from build123d import *

# Parameters (mm, degrees)
SKETCH016_R            = 4.25
PAD015_DEPTH           = 30
PAD014_DEPTH           = 3
PRISM008_DEPTH         = 10
PRISM008_ROLL_ANGLE    = 90
PAD011_DEPTH           = 15
SKETCH010_R            = 1
PAD010_DEPTH           = 22.5
CYLINDER017_R          = 4.25
CYLINDER017_DEPTH      = 10
CYLINDER016_R          = 5.25
CYLINDER016_DEPTH      = 10
CYLINDER014_R          = 1.75
CYLINDER014_DEPTH      = 36
CYLINDER014_ROLL_ANGLE = -90
PAD004_DEPTH           = 5
CHAMFER002_SIZE        = 1
CYLINDER012_R          = 1.75
CYLINDER012_DEPTH      = 11
CYLINDER012_ROLL_ANGLE = 90
CYLINDER013_R          = 5.5
CYLINDER013_DEPTH      = 14
CYLINDER013_ROLL_ANGLE = -90
BOX010_W               = 35
BOX010_H               = 60
BOX010_DEPTH           = 35
PAD003_DEPTH           = 42
FILLET002_R            = 0.5
CHAMFER003_SIZE        = 1
CHAMFER006_SIZE        = 2
CHAMFER007_SIZE        = 1


with BuildPart() as pad015:
    # Sketch016 → Pad015 (new body)
    with BuildSketch(Plane(origin=(23.25, 34, -10), x_dir=(-0.996195, -0.087156, 0), z_dir=(0, 0, 1))):
        with Locations((47, 7)):
            Circle(SKETCH016_R)
    extrude(amount=PAD015_DEPTH)


with BuildPart() as fusion011:
    # Sketch014 → Pad014 (new body)
    with BuildSketch(Plane(origin=(23.25, 34, -10), x_dir=(-0.996195, -0.087156, 0), z_dir=(0, 0, 1))):
        with BuildLine():
            ThreePointArc((49.709474, 10.274332), (43.52198, 9.442514), (44.839693, 3.340003))
            Line((44.839693, 3.340003), (61.15095, -6.287705))
            ThreePointArc((61.15095, -6.287705), (64.799282, -5.499923), (64.301984, -1.800786))
            Line((49.709474, 10.274332), (64.301984, -1.800786))
        make_face()
    extrude(amount=PAD014_DEPTH)

    # Fusion011: union Pad015
    add(pad015.part)


with BuildPart() as fake_axis_nut_room:
    # Prism008 → Prism008 (new body)
    with BuildSketch(Plane.XY):
        Polygon((3.2, 0), (1.6, 2.771281), (-1.6, 2.771281), (-3.2, 0), (-1.6, -2.771281), (1.6, -2.771281), align=None)
    extrude(amount=PRISM008_DEPTH)


with BuildPart() as fake_axis_nut_room_1:
    # Prism008 roll: moved
    add(fake_axis_nut_room.part.rotate(Axis((0, 0, 0), (1, 0, 0)), PRISM008_ROLL_ANGLE))


with BuildPart() as fake_axis_nut_room_2:
    # Prism008 placement: moved
    add(fake_axis_nut_room_1.part.moved(Location((-47, 25.5, 7))))


with BuildPart() as pad011:
    # Sketch011 → Pad011 (new body)
    with BuildSketch(Plane(origin=(0, 0, -10), x_dir=(1, 0, 0), z_dir=(0, 0, -1))):
        with BuildLine():
            ThreePointArc((-48.5, -22.8), (-50.7, -25), (-48.5, -27.2))
            Line((-48.5, -27.2), (-39.5, -27.2))
            ThreePointArc((-39.5, -27.2), (-37.3, -25), (-39.5, -22.8))
            Line((-48.5, -22.8), (-39.5, -22.8))
        make_face()
    extrude(amount=-PAD011_DEPTH)


with BuildPart() as pad010:
    # Sketch010 → Pad010 (new body)
    with BuildSketch(Plane(origin=(0, 41, 0), x_dir=(-1, 0, 0), z_dir=(0, 1, 0))):
        with Locations((43.25, 26.75)):
            Circle(SKETCH010_R)
        with Locations((50.75, 26.75)):
            Circle(SKETCH010_R)
        with Locations((43.25, -1.25)):
            Circle(SKETCH010_R)
        with Locations((50.75, -1.25)):
            Circle(SKETCH010_R)
        with Locations((47, -1.25)):
            Circle(SKETCH010_R)
        with Locations((47, 26.75)):
            Circle(SKETCH010_R)
        Polygon((40.5, 24.5), (53.5, 24.5), (53.5, 1), (40.5, 1), (30.5, 1), (30.5, 24.5), align=None)
    extrude(amount=-PAD010_DEPTH)


with BuildPart() as cylinder017:
    # Cylinder017 → Cylinder017 (new body)
    with BuildSketch(Plane.XY.offset(-5)):
        Circle(CYLINDER017_R)
    extrude(amount=CYLINDER017_DEPTH)


with BuildPart() as fusion008:
    # Cylinder016 → Cylinder016 (new body)
    with BuildSketch(Plane.XY):
        Circle(CYLINDER016_R)
    extrude(amount=CYLINDER016_DEPTH)

    # Fusion008: union Cylinder017
    add(cylinder017.part)


with BuildPart() as fusion008_1:
    # Fusion008 placement: moved
    add(fusion008.part.moved(Location((-23, 23, 32))))


with BuildPart() as cilindro014:
    # Cylinder014 → Cylinder014 (new body)
    with BuildSketch(Plane.XY):
        Circle(CYLINDER014_R)
    extrude(amount=CYLINDER014_DEPTH)


with BuildPart() as cilindro014_1:
    # Cylinder014 roll: moved
    add(cilindro014.part.rotate(Axis((0, 0, 0), (1, 0, 0)), CYLINDER014_ROLL_ANGLE))


with BuildPart() as cilindro014_2:
    # Cylinder014 placement: moved
    add(cilindro014_1.part.moved(Location((-59, 8, 29))))


with BuildPart() as pad004:
    # Sketch004 → Pad004 (new body)
    with BuildSketch(Plane(origin=(0, 14, 0), x_dir=(-1, 0, 0), z_dir=(0, 1, 0))):
        with BuildLine():
            ThreePointArc((61.828427, 26.171573), (62.695518, 30.530734), (59, 33))
            Line((59, 33), (54, 33))
            Line((54, 33), (54, 18.343146))
            Line((54, 18.343146), (61.828427, 26.171573))
        make_face()
    extrude(amount=PAD004_DEPTH)


with BuildPart() as chamfer002:
    # Clone006 base: copy of Pad004
    add(pad004.part)


with BuildPart() as chamfer002_1:
    # Clone006 placement: moved
    add(chamfer002.part.moved(Location((0, 19, 0))))

    # Fusion006: union Pad004
    add(pad004.part)

    # Chamfer002
    chamfer002_edges = [chamfer002_1.edges().sort_by_distance(p)[0] for p in [
        (-62.695518, 14, 30.530734),
        (-62.695518, 38, 30.530734),
    ]]
    chamfer(chamfer002_edges, length=CHAMFER002_SIZE)


with BuildPart() as cilindro012:
    # Cylinder012 → Cylinder012 (new body)
    with BuildSketch(Plane.XY):
        Circle(CYLINDER012_R)
    extrude(amount=CYLINDER012_DEPTH)


with BuildPart() as cilindro012_1:
    # Cylinder012 roll: moved
    add(cilindro012.part.rotate(Axis((0, 0, 0), (1, 0, 0)), CYLINDER012_ROLL_ANGLE))


with BuildPart() as cilindro012_2:
    # Cylinder012 placement: moved
    add(cilindro012_1.part.moved(Location((-47, 23, 7))))


with BuildPart() as cilindro013:
    # Cylinder013 → Cylinder013 (new body)
    with BuildSketch(Plane.XY):
        Circle(CYLINDER013_R)
    extrude(amount=CYLINDER013_DEPTH)


with BuildPart() as cilindro013_1:
    # Cylinder013 roll: moved
    add(cilindro013.part.rotate(Axis((0, 0, 0), (1, 0, 0)), CYLINDER013_ROLL_ANGLE))


with BuildPart() as cilindro013_2:
    # Cylinder013 placement: moved
    add(cilindro013_1.part.moved(Location((-59, 19, 29))))


with BuildPart() as cubo010:
    # Box010 → Box010 (new body)
    with BuildSketch(Plane(origin=(-41, 0, -5), x_dir=(1, 0, 0), z_dir=(0, 0, 1))):
        with Locations((17.5, 30)):
            Rectangle(BOX010_W, BOX010_H)
    extrude(amount=BOX010_DEPTH)


with BuildPart() as bracket:
    # Sketch003 → Pad003 (new body)
    with BuildSketch(Plane.XY.offset(-9)):
        with BuildLine():
            ThreePointArc((-22.999967, 14), (-14.106152, 21.621786), (-20.276052, 31.577885))
            Line((-40.499967, 38), (-20.276052, 31.577885))
            Line((-55.999967, 38), (-40.499967, 38))
            Line((-55.999967, 14), (-55.999967, 38))
            Line((-22.999967, 14), (-55.999967, 14))
        make_face()
    extrude(amount=PAD003_DEPTH)

    # Cut007: cut Cubo010
    add(cubo010.part, mode=Mode.SUBTRACT)

    # Cut008: cut Cilindro013
    add(cilindro013_2.part, mode=Mode.SUBTRACT)

    # Fillet002
    fillet002_edges = [bracket.edges().sort_by_distance(p)[0] for p in [
        (-55.999967, 26, 24.390249),
        (-55.225083, 26, 33),
    ]]
    fillet(fillet002_edges, radius=FILLET002_R)

    # Chamfer003
    chamfer003_edges = [bracket.edges().sort_by_distance(p)[0] for p in [
        (-55.999967, 14, 12),
        (-55.999967, 26, -9),
        (-55.999967, 38, 12),
        (-39.499967, 14, 33),
        (-14.106152, 21.621786, 33),
        (-48.249967, 38, 33),
        (-48.249967, 38, -9),
    ]]
    chamfer(chamfer003_edges, length=CHAMFER003_SIZE)

    # Cut010: cut Cilindro012
    add(cilindro012_2.part, mode=Mode.SUBTRACT)

    # Fusion007: union Chamfer002
    add(chamfer002_1.part)

    # Cut011: cut Cilindro014
    add(cilindro014_2.part, mode=Mode.SUBTRACT)

    # Cut012: cut Fusion008
    add(fusion008_1.part, mode=Mode.SUBTRACT)

    # Cut015: cut Pad010
    add(pad010.part, mode=Mode.SUBTRACT)

    # Chamfer006
    chamfer006_edges = [bracket.edges().sort_by_distance(p)[0] for p in [
        (-41, 28.25, 1),
    ]]
    chamfer(chamfer006_edges, length=CHAMFER006_SIZE)

    # Cut016: cut Pad011
    add(pad011.part, mode=Mode.SUBTRACT)

    # Chamfer007
    chamfer007_edges = [bracket.edges().sort_by_distance(p)[0] for p in [
        (-14.106152, 21.621786, -9),
    ]]
    chamfer(chamfer007_edges, length=CHAMFER007_SIZE)

    # Cut017: cut fake_axis_nut_room
    add(fake_axis_nut_room_2.part, mode=Mode.SUBTRACT)

    # Cut020: cut Fusion011
    add(fusion011.part, mode=Mode.SUBTRACT)


solid = bracket.part
Source: CAD feature listing. Evaluate the final solid. Frame: model axes, mm. A direction names the side the tool comes from. Coordinates: 2 decimals unless noted, no trailing zeros. Loops run counter-clockwise (first coordinate to the right, second up) from the corner with the lowest first, then second, coordinate; pieces in that order, holes last. Notation, with made-up numbers: M 65.25,-39 L 73.25,-39 A9 ccw 73.25,-26 Z; hole C -1.5,-1.5 d11. An arc over 180 degrees is marked long. Answer in a Markdown table with one row per item.
Q1. First-contact query: pin 1 (4 mm diameter, centred on x = -47, z = 7, fed in from +Y); pin 2 (8 mm diameter, centred on y = 23, z = -0.5, fed in from +X); pin 3 (10 mm diameter, centred on y = 26, z = 9, fed in from +X). Flat tips, straight axial feed; report the tip coordinate or a pass-through.
Answers below:
| item | result |
|---|---|
| pin 1 | stops at y = 15.5 |
| pin 2 | stops at x = -41 |
| pin 3 | stops at x = -53.5 |
Q2. Ray query, probe 1 along Z at (x, y) = (-50.75, 34.25); probe 2 along Z at (x, y) = (-32, 27.25); probe 3 along Z at (x, y) = (-35.5, 22.25). Return the intervals inside material, ascending. Write a range as from..to.
Answers below:
| item | result |
|---|---|
| probe 1 | z = -9..-2.25, -0.25..1, 24.5..25.75, 27.75..33 |
| probe 2 | z = -7..-5, 30..33 |
| probe 3 | z = -9..-5, 30..33 |
Q3. Draft query along X for faces 6 (the flat face through (-30.53, 34.834, -6.521)), 7 (the flat face through (-33.06, 24.736, -8.014)), 8 (the flat face through (-57, 19, 28)). Return one class per face: pulls with the +X half, pulls with the -X half, needs draft (parallel to the pull), parting line crosses it, or undercut.
Answers below:
| item | result |
|---|---|
| face 6 | pulls with the +X half |
| face 7 | undercut |
| face 8 | needs draft |
Q4. Set-up query: faces 1 (the flat face through (-58.873, 16.972, 23.217)), 2 (the flat face through (-53.5, 28, 13)), 3 (the flat face through (-30.53, 34.834, 30.986)), 4 (the cylindrical face through (-41.753, 33.881, -8.014)), 5 (the flat face through (-44.611, 17.021, 5.595)). Return all of +Z, -Z, +X, -X, +Y, -Y with unobstructed straight access to the full face (end or side cutting, diameter ignored); none if empty.
Answers below:
| item | result |
|---|---|
| face 1 | -Z, -X, +Y, -Y |
| face 2 | +X, +Y |
| face 3 | +Z, -Z, +X, +Y |
| face 4 | -Z |
| face 5 | +Y |
Q5. Section C-C on z = 14. Return the cut outline in (x, y), plus the area to 3 significant figures.
Answers below:
| item | result |
|---|---|
| outline | M -56,15 L -55,14 L -41,14 L -41,18.5 L -53.5,18.5 L -53.5,38 L -55,38 L -56,37 Z |
| area | 115 mm^2 |
Q6. Section B-B on y = 34.25. State how many separate pieces and enclosed holes the cut face has, plus the area to 3 significant figures.
Answers below:
| item | result |
|---|---|
| separate pieces | 1 |
| enclosed holes | 7 |
| area | 439 mm^2 |
Q7. Section A-A on z = 29. Return the cut outline in (x, y).
Answers below:
| item | result |
|---|---|
| outline | M -63,15 L -62,14 L -60.75,14 L -60.75,19 L -63,19 Z; M -63,33 L -60.75,33 L -60.75,38 L -62,38 L -63,37 Z; M -57.25,14 L -41,14 L -41,38 L -57.25,38 L -57.25,33 L -53.5,33 L -53.5,19 L -57.25,19 Z |
